Can you work these out from the model? Positions are in its coordinate system, mm. Face numbers are marked on the shaded views. A direction names the side the tool comes from. Give positions to 0.01 mm unless a question says otherwise; leave off trailing zeros. Order: outer loops, then holes, each group sorted by start corner. A loop starts at its lowest first (then second) coordinate and runs counter-clockwise, first axis right, second up. Notation, with made-up numbers: (5, 65) - (57, 65) arc R22 ccw to (57, 88) - close; hole circle Ø2 at (-37, 57.25). An arc over 180 degrees is marked (long way). Answer as a JSON object with one key per item and string values.
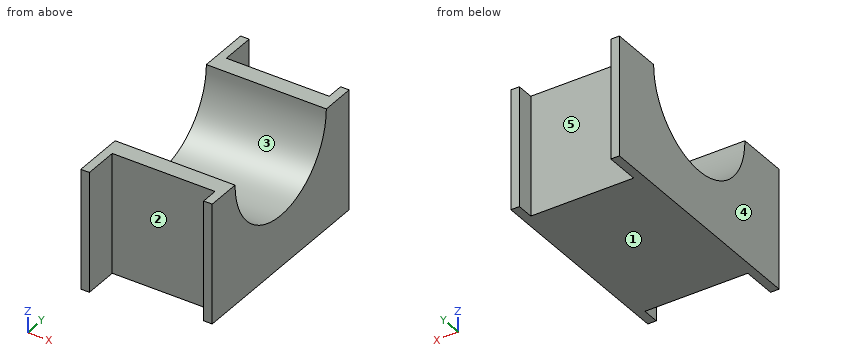
```python
from build123d import *

# Parameters (mm, degrees)
ESQUISSE1_W             = 3.5
ESQUISSE1_H             = 7
BOSS_EXTRU_1_DEPTH      = 3.5
ESQUISSE2_W             = 3
ESQUISSE2_H             = 3.5
ENL_V_MAT_EXTRU_1_DEPTH = 1
ESQUISSE3_W             = 3
ESQUISSE3_H             = 3.5
ENL_V_MAT_EXTRU_2_DEPTH = 1
ENL_V_MAT_EXTRU_4_DEPTH = 10
ESQUISSE6_W             = 3.5
ESQUISSE6_H             = 0.5
ENL_V_MAT_EXTRU_5_DEPTH = 2


with BuildPart() as part:
    # Esquisse1 → Boss.-Extru.1 (new body)
    with BuildSketch(Plane.XY):
        with Locations((0.25, 0)):
            Rectangle(ESQUISSE1_W, ESQUISSE1_H)
    extrude(amount=BOSS_EXTRU_1_DEPTH)

    # Esquisse2 → Enlèv. mat.-Extru.1 (cut)
    with BuildSketch(Plane(origin=(0, 3.5, 0), x_dir=(1, 0, 0), z_dir=(0, 1, 0))):
        with Locations((0.25, -1.75)):
            Rectangle(ESQUISSE2_W, ESQUISSE2_H)
    extrude(amount=-ENL_V_MAT_EXTRU_1_DEPTH, mode=Mode.SUBTRACT)

    # Esquisse3 → Enlèv. mat.-Extru.2 (cut)
    with BuildSketch(Plane(origin=(0, -3.5, 0), x_dir=(-1, 0, 0), z_dir=(0, -1, 0))):
        with Locations((-0.25, -1.75)):
            Rectangle(ESQUISSE3_W, ESQUISSE3_H)
    extrude(amount=-ENL_V_MAT_EXTRU_2_DEPTH, mode=Mode.SUBTRACT)

    # Esquisse5 → Enlèv. mat.-Extru.4 (cut)
    with BuildSketch(Plane(origin=(2, 0, 0), x_dir=(0, 0, -1), z_dir=(1, 0, 0))):
        with BuildLine():
            Line((-3.5, -2), (-3.5, 2))
            ThreePointArc((-3.5, 2), (-1.5, 0), (-3.5, -2))
        make_face()
    extrude(amount=-ENL_V_MAT_EXTRU_4_DEPTH, mode=Mode.SUBTRACT)

    # Esquisse6 → Enlèv. mat.-Extru.5 (cut)
    with BuildSketch(Plane(origin=(2, 0, 0), x_dir=(0, 0, -1), z_dir=(1, 0, 0))):
        with Locations((-1.75, 3.25)):
            Rectangle(ESQUISSE6_W, ESQUISSE6_H)
        with Locations((-1.75, -3.25)):
            Rectangle(ESQUISSE6_W, ESQUISSE6_H)
    extrude(amount=-ENL_V_MAT_EXTRU_5_DEPTH, mode=Mode.SUBTRACT)


solid = part.part
```
Q1. Which directions (+Z, -Z, +X, -X, +Y, -Y) give clear straight access to the entire face, cutting with the end or side of a thin tool? Please do the marked faces 1 and 2.
Recorded:
{"face 1": "-Z, +X, -X, +Y, -Y", "face 2": "+Z, -Z, -Y"}
Q2. We'd pull the mould along X, two halves only. Please class the marked faces 3, 4 and 5: released by +X, released by -X, zero draft, split by the parting line, or undercut.
Recorded:
{"face 3": "zero draft", "face 4": "released by -X", "face 5": "undercut"}
Q3. I'm going to push a flat-ended pin straight in: pin 1 Ø2 at (x, z) = (0.5, 2.5) entering from -Y. Where does the tip first touch, or does it pass through?
Recorded:
{"pin 1": "stops at y = -2.5"}
Q4. If we section it at C-C, the plane x = 0.2: Please give me the cut outline in (y, z), then the cut area to 3 significant figures.
Recorded:
{"outline": "(-2.5, 0) - (2.5, 0) - (2.5, 3.5) - (2, 3.5) arc R2 cw to (-2, 3.5) - (-2.5, 3.5) - close", "area": "11.2 mm^2"}
Q5. If we section it at A-A, the plane y = -2.75: Please give me the cut outline in (x, z), then the cut area to 3 significant figures.
Recorded:
{"outline": "(-1.5, 0) - (-1.25, 0) - (-1.25, 3.5) - (-1.5, 3.5) - close; (1.75, 0) - (2, 0) - (2, 3.5) - (1.75, 3.5) - close", "area": "1.75 mm^2"}
Q6. If we section it at D-D, the plane y = 0: Please give me the cut outline in (x, z).
Recorded:
{"outline": "(-1.5, 0) - (2, 0) - (2, 1.5) - (-1.5, 1.5) - close"}
Q7. If we section it at B-B, the plane z = 1.7: Please give me the cut outline in (x, y), then the cut area to 3 significant figures.
Recorded:
{"outline": "(-1.5, -3.5) - (-1.25, -3.5) - (-1.25, -2.5) - (1.75, -2.5) - (1.75, -3) - (2, -3) - (2, -0.87) - (-1.5, -0.87) - close; (-1.5, 0.87) - (2, 0.87) - (2, 3) - (1.75, 3) - (1.75, 2.5) - (-1.25, 2.5) - (-1.25, 3.5) - (-1.5, 3.5) - close", "area": "12.1 mm^2"}
Q8. I need wall thicknesses on L1, parallel to X at y = 2.75, z = 2.1; L2, parallel to Y at x = -1.2, z = 0.5; L3, parallel to Y at x = -0.65, z = 2.1. Which ranges of each line are inside material? Lowest first, please.
Recorded:
{"L1": "x = -1.5 to -1.25, 1.75 to 2", "L2": "y = -2.5 to 2.5", "L3": "y = -2.5 to -1.43, 1.43 to 2.5"}
